Geometry check sheet. Reference: drawing and pictorial views, mm from the part's lowest x, y, z. A direction names the side the tool comes from. Give positions to 0.01 mm unless a question says otherwise; leave off trailing zeros. Loops run counter-clockwise (first coordinate to the right, second up) from the corner with the lowest first, then second, coordinate; pieces in that order, holes last. Notation, with made-up numbers: (23.5, 58) - (82.5, 58) arc R12 ccw to (82.5, 75) - close; hole circle Ø7 at (60.5, 0.25). An arc over 180 degrees is marked (long way). Use CSV: the item, a comma, the result in double quotes.
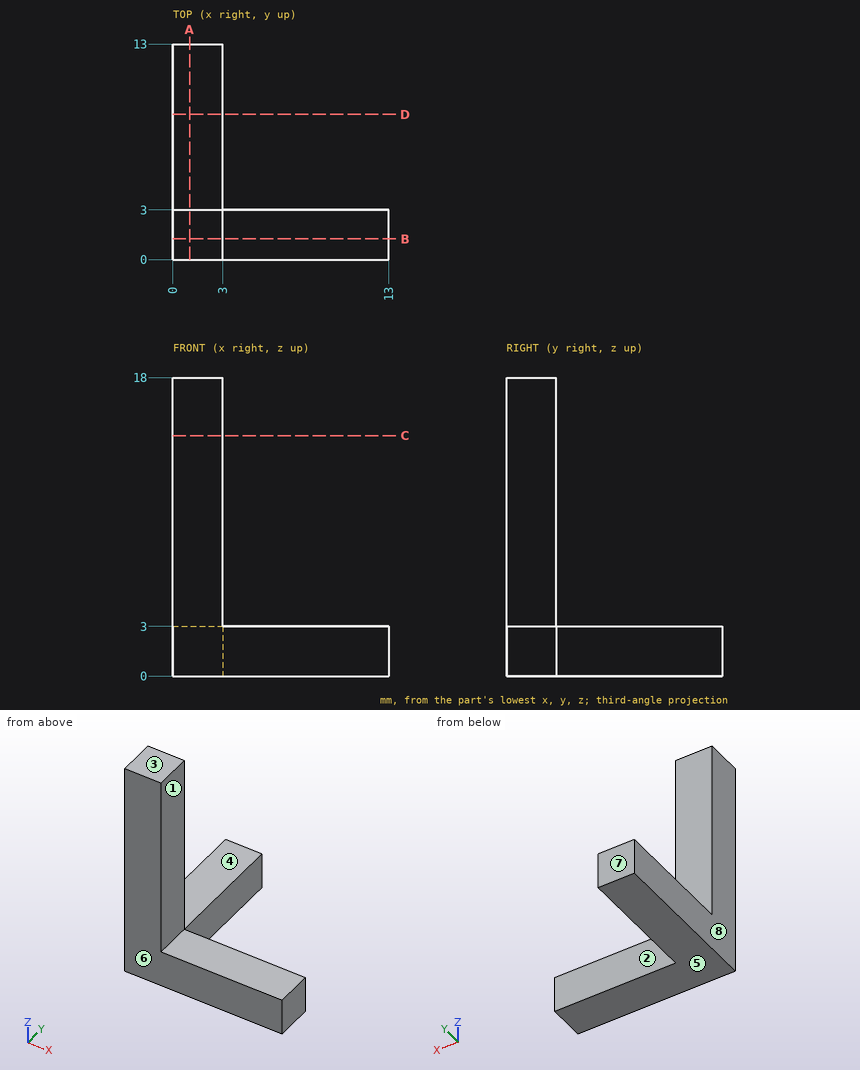
1. Go/stop test with flat-tipped pins: pin 1 Ø3.5 at (x, y) = (2, 9.5) entering from +Z; pin 2 Ø3.5 at (x, z) = (5.5, 1) entering from +Y; pin 3 Ø3.5 at (y, z) = (1, 10) entering from +X. Record where each tip stops, or that it passes through.
Completed:
pin 1,"stops at z = 3"
pin 2,"stops at y = 3"
pin 3,"stops at x = 3"
2. Sectioned sample at A-A, the plane x = 1. Record the boundary of the cut face in (y, z), and give its area (3 significant figures).
Completed:
outline,"(0, 0) - (13, 0) - (13, 3) - (3, 3) - (3, 18) - (0, 18) - close"
area,"84.0 mm²"
3. Set-up check for the marked faces 1, 2, 3, 4 and 5: record each of +Z, -Z, +X, -X, +Y, -Y from which the full face is reachable in a straight line by a thin tool's end or side.
Completed:
face 1,"+Z, +X, +Y, -Y"
face 2,"+Z, -Z, +X, +Y"
face 3,"+Z, +X, -X, +Y, -Y"
face 4,"+Z, +X, -X, +Y"
face 5,"-Z, +X, -X, +Y, -Y"
4. Sectioned sample at C-C, the plane z = 14.5. Record the boundary of the cut face in (x, y), and give its area (3 significant figures).
Completed:
outline,"(0, 0) - (3, 0) - (3, 3) - (0, 3) - close"
area,"9.00 mm²"
5. Release check for a two-part mould opening along Y. For the marked faces 6, 7 and 8 record: released by +Y, released by -Y, zero draft, split by the parting line, or undercut.
Completed:
face 6,"released by -Y"
face 7,"released by +Y"
face 8,"zero draft"
6. Scan line: line 1 along Z through (x, y) = (3.5, 1.25). Record every from-to range of solid material in increasing order.
Completed:
line 1,"z = 0 to 3"
